Work out the finished part from the listing and answer in its coordinate system (mm). Round coordinates to 2 decimals unless told otherwise and drop trailing zeros. Loops run counter-clockwise (first coordinate to the right, second up) from the corner with the lowest first, then second, coordinate; pieces in that order, holes last. Notation, with made-up numbers: M 4.25,53.25 L 61.25,53.25 A7 ccw 61.25,61.25 Z; hole C -18,-19 d9. An arc over 180 degrees is marked long. One line per item, written item: value.
```python
from build123d import *

# Parameters (mm, degrees)
SKETCH2_R           = 6.35
SKETCH2_W           = 2.794
SKETCH2_H           = 25.4
BOSS_EXTRUDE1_DEPTH = 2.794


with BuildPart() as part:
    # Sketch2 → Boss-Extrude1 (new body)
    with BuildSketch(Plane(origin=(0, 0, 0), x_dir=(1, 0, 0), z_dir=(0, 1, 0))):
        Polygon((0, 0), (25.4, 0), (25.4, -2.794), (40.64, -2.794), (40.64, 0), (99.06, 0), (99.06, -2.794), (114.3, -2.794), (114.3, 0), (139.7, 0), (139.7, 67.31), (114.3, 67.31), (114.3, 70.104), (99.06, 70.104), (99.06, 67.31), (40.64, 67.31), (40.64, 70.104), (25.4, 70.104), (25.4, 67.31), (0, 67.31), align=None)
        with Locations((20.574, 33.655)):
            Circle(SKETCH2_R, mode=Mode.SUBTRACT)
        with Locations((131.191, 33.655)):
            Rectangle(SKETCH2_W, SKETCH2_H, mode=Mode.SUBTRACT)
    extrude(amount=BOSS_EXTRUDE1_DEPTH)


solid = part.part
```
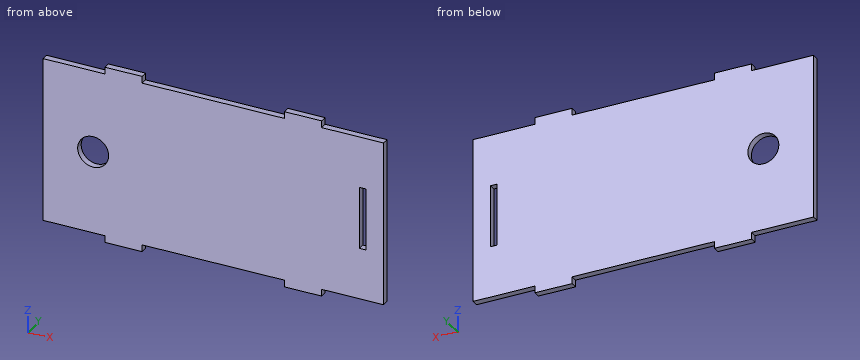
1) Find section A-A (z = -24). Give the vertices of the cut face in (x, y), then the cut area to 3 significant figures.
Check values:
outline: M 0,0 L 129.79,0 L 129.79,2.79 L 0,2.79 Z; M 132.59,0 L 139.7,0 L 139.7,2.79 L 132.59,2.79 Z
area: 383 mm2
2) Find the intervals of material crossed by probe 1 along X at (y, z) = (1.3, -34.5); probe 2 along X at (y, z) = (1.55, -31.5); probe 3 along X at (y, z) = (0.35, -27), in increasing order. Write a range as from..to.
Check values:
probe 1: 0..14.28, 26.87..129.79, 132.59..139.7
probe 2: 0..14.6, 26.55..129.79, 132.59..139.7
probe 3: 0..129.79, 132.59..139.7
3) Find section D-D (x = 61.5). Give the vertices of the cut face in (y, z).
Check values:
outline: M 0,-67.31 L 2.79,-67.31 L 2.79,0 L 0,0 Z
4) Each of these flat-tipped pins is pushed along its axis until it touches: pin 1 (0.8 mm diameter, centred on x = 18, y = 1.5, fed in from +Z); pin 2 (1.4 mm diameter, centred on y = 1.5, z = 2, fed in from -X); pin 3 (1.4 mm diameter, centred on x = 70.5, y = 1, fed in from -Z). Where does it stop, or does it pass through?
Check values:
pin 1: z = 0
pin 2: x = 25.4
pin 3: z = -67.31
5) Find section B-B (x = 15.5). Give the vertices of the cut face in (y, z), then the cut area to 3 significant figures.
Check values:
outline: M 0,-67.31 L 2.79,-67.31 L 2.79,-37.47 L 0,-37.47 Z; M 0,-29.84 L 2.79,-29.84 L 2.79,0 L 0,0 Z
area: 167 mm2
6) Find section C-C (y = 1.65). Give the vertices of the cut face in (x, z) (3 decimals).
Check values:
outline: M 0,-67.31 L 25.4,-67.31 L 25.4,-70.104 L 40.64,-70.104 L 40.64,-67.31 L 99.06,-67.31 L 99.06,-70.104 L 114.3,-70.104 L 114.3,-67.31 L 139.7,-67.31 L 139.7,0 L 114.3,0 L 114.3,2.794 L 99.06,2.794 L 99.06,0 L 40.64,0 L 40.64,2.794 L 25.4,2.794 L 25.4,0 L 0,0 Z; hole C 20.574,-33.655 d12.7; hole M 129.794,-46.355 L 132.588,-46.355 L 132.588,-20.955 L 129.794,-20.955 Z
